The listing builds one solid part. Answer for the finished solid, in the listing's coordinates (mm). A direction names the side the tool comes from. Round coordinates to 2 decimals unless told otherwise and drop trailing zeros. Write each loop counter-clockwise with the first axis right and the second up, starting at its lowest first coordinate (ties: lowest second). Pieces come first, ordered by that corner, then holes.
from build123d import *

# Parameters (mm, degrees)
SKETCH004_R   = 1.5
PAD004_DEPTH  = 48
SKETCH005_R   = 11
SKETCH005_R_2 = 6.5
PAD005_DEPTH  = 2
SKETCH006_R   = 2.5
PAD006_DEPTH  = 24


with BuildPart() as part:
    # Sketch004 → Pad004 (new body)
    with BuildSketch(Plane.XY):
        Polygon((-21.15, 17.15), (-21.15, -17.15), (-17.15, -21.15), (17.15, -21.15), (21.15, -17.15), (21.15, 17.15), (17.15, 21.15), (-17.15, 21.15), align=None)
        with Locations((-15.5, 15.5)):
            Circle(SKETCH004_R, mode=Mode.SUBTRACT)
        with Locations((15.5, 15.5)):
            Circle(SKETCH004_R, mode=Mode.SUBTRACT)
        with Locations((15.5, -15.5)):
            Circle(SKETCH004_R, mode=Mode.SUBTRACT)
        with Locations((-15.5, -15.5)):
            Circle(SKETCH004_R, mode=Mode.SUBTRACT)
    extrude(amount=-PAD004_DEPTH)

    # Sketch005 (on Face13 of Pad004) → Pad005 (join)
    with BuildSketch(Plane.XY):
        Circle(SKETCH005_R)
        Circle(SKETCH005_R_2, mode=Mode.SUBTRACT)
    extrude(amount=PAD005_DEPTH)

    # Sketch006 (on Face18 of Pad005) → Pad006 (join)
    with BuildSketch(Plane.XY):
        Circle(SKETCH006_R)
    extrude(amount=PAD006_DEPTH)


solid = part.part
1. Section A-A on y = 15.5 is taken. Determine the outline of the cut face in (x, z).
Geometry says:
outline: (-21.15, -48) - (-17, -48) - (-17, 0) - (-21.15, 0) - close; (-14, -48) - (14, -48) - (14, 0) - (-14, 0) - close; (17, -48) - (21.15, -48) - (21.15, 0) - (17, 0) - close
2. Section D-D on x = -9 is taken. Determine the outline of the cut face in (y, z), plus the area to 3 significant figures.
Geometry says:
outline: (-21.15, -48) - (21.15, -48) - (21.15, 0) - (6.32, 0) - (6.32, 2) - (-6.32, 2) - (-6.32, 0) - (-21.15, 0) - close
area: 2,060 mm2
3. Straight lines are drawn through the part: line 1 along Y through (x, z) = (15.5, -22.5); line 2 along Y through (x, z) = (15, -35). For each, find the intervals that lie inside material, in ascending order.
Geometry says:
line 1: y = -21.15 to -17, -14 to 14, 17 to 21.15
line 2: y = -21.15 to -16.91, -14.09 to 14.09, 16.91 to 21.15
4. Given pin 1 (1.8 mm diameter, centred on x = -15.5, y = -15.5, fed in from -Z); pin 2 (4 mm diameter, centred on x = 16, y = -6.5, fed in from +Z); pin 3 (5 mm diameter, centred on x = 15.5, y = 15.5, fed in from -Z); pin 4 (3 mm diameter, centred on x = -6.5, y = 6.5, fed in from +Z), each flat-ended and moving along its own axis, determine where each tip first touches the part or whether it passes through.
Geometry says:
pin 1: passes through
pin 2: stops at z = 0
pin 3: stops at z = -48
pin 4: stops at z = 2
5. For a pull along X with two mould halves and no side action, classify faces 3 (the face through (-19.2, -19.1, -23.7)), 4 (the face through (0, 0, -48)), 5 (the face through (14, -15.43, -23.66)) as released by +X, released by -X, zero draft, split by the parting line, or undercut.
Geometry says:
face 3: released by -X
face 4: zero draft
face 5: undercut
6. Section C-C on z = -13 is taken. Determine the outline of the cut face in (x, y), plus the area to 3 significant figures.
Geometry says:
outline: (-21.15, -17.15) - (-17.15, -21.15) - (17.15, -21.15) - (21.15, -17.15) - (21.15, 17.15) - (17.15, 21.15) - (-17.15, 21.15) - (-21.15, 17.15) - close; hole circle Ø3 at (-15.5, -15.5); hole circle Ø3 at (-15.5, 15.5); hole circle Ø3 at (15.5, -15.5); hole circle Ø3 at (15.5, 15.5)
area: 1,730 mm2
7. A tool of negligible diameter and unlimited length cuts with its end or side. For faces 1 (the face through (-5.158, -3.955, 0.986)), 2 (the face through (-21.15, 0, -24)), from which of +Z, -Z, +X, -X, +Y, -Y can it reach the whole face along a straight path? Write none if from no direction.
Geometry says:
face 1: +Z
face 2: +Z, -Z, -X, +Y, -Y
